For this review, take the finished solid that the model builds, in its own axes (mm). A direction names the side the tool comes from. Round coordinates to 2 decimals unless told otherwise and drop trailing zeros. Write each loop counter-clockwise with the first axis right and the second up, starting at its lowest first coordinate (ties: lowest second). Pieces come first, ordered by that corner, then holes. Notation, with made-up numbers: M 79,65.5 L 128,65.5 A33 ccw 128,97.5 Z; hole C 85.5,11 d2. An arc over 180 degrees is marked long. Answer in a Markdown table with one row per item.
```python
from build123d import *

# Parameters (mm, degrees)
SKETCH1_R           = 2.5
BOSS_EXTRUDE1_DEPTH = 2.5


with BuildPart() as part:
    # Sketch1 → Boss-Extrude1 (new body)
    with BuildSketch(Plane(origin=(0, 0, -1.25), x_dir=(-1, 0, 0), z_dir=(0, 0, -1))):
        with BuildLine():
            Line((-1.337750611, -12.7), (75.946, -12.7))
            Line((75.946, -12.7), (82.296, -6.35))
            Line((82.296, -6.35), (82.296, 6.35))
            Line((82.296, 6.35), (75.946, 12.7))
            Line((75.946, 12.7), (57.193204579, 12.7))
            ThreePointArc((57.193204579, 12.7), (55.429269089, 13.235083981), (54.259887063, 14.659980102))
            Line((54.259887063, 14.659980102), (48.733705431, 28.001362746))
            ThreePointArc((48.733705431, 28.001362746), (48.553029681, 29.835794416), (49.421958916, 31.461446674))
            Line((49.421958916, 31.461446674), (62.682187725, 44.721675483))
            Line((62.682187725, 44.721675483), (62.682187725, 53.701931604))
            Line((62.682187725, 53.701931604), (53.701931604, 62.682187725))
            Line((53.701931604, 62.682187725), (44.721675483, 62.682187725))
            Line((44.721675483, 62.682187725), (-9.92618865, 8.034323593))
            Line((-9.92618865, 8.034323593), (-1.337750611, -12.7))
        make_face()
        with Locations((12.7, 0)):
            Circle(SKETCH1_R, mode=Mode.SUBTRACT)
        with Locations((25.4, 0)):
            Circle(SKETCH1_R, mode=Mode.SUBTRACT)
        with Locations((38.1, 0)):
            Circle(SKETCH1_R, mode=Mode.SUBTRACT)
        with Locations((50.8, 0)):
            Circle(SKETCH1_R, mode=Mode.SUBTRACT)
        Circle(SKETCH1_R, mode=Mode.SUBTRACT)
        with Locations((76.2, 0)):
            Circle(SKETCH1_R, mode=Mode.SUBTRACT)
        with Locations((63.5, 0)):
            Circle(SKETCH1_R, mode=Mode.SUBTRACT)
        with Locations((53.881536726, 53.881536726)):
            Circle(SKETCH1_R, mode=Mode.SUBTRACT)
        with Locations((44.901280605, 44.901280605)):
            Circle(SKETCH1_R, mode=Mode.SUBTRACT)
        with Locations((35.921024484, 35.921024484)):
            Circle(SKETCH1_R, mode=Mode.SUBTRACT)
        with Locations((26.940768363, 26.940768363)):
            Circle(SKETCH1_R, mode=Mode.SUBTRACT)
        with Locations((17.960512242, 17.960512242)):
            Circle(SKETCH1_R, mode=Mode.SUBTRACT)
        with Locations((8.980256121, 8.980256121)):
            Circle(SKETCH1_R, mode=Mode.SUBTRACT)
    extrude(amount=-BOSS_EXTRUDE1_DEPTH)


solid = part.part
```
Q1. For probe 1 along Y at (x, z) = (-25.4, 0.7); probe 2 along Y at (x, z) = (-7.5, 0.1); probe 3 along Y at (x, z) = (-46, 0.05), list the stretches that pass through material, from the lowest coordinate up.
Found:
| item | result |
|---|---|
| probe 1 | -12.7 to -2.5, 2.5 to 24.97, 28.91 to 43.36 |
| probe 2 | -12.7 to 6.97, 10.99 to 25.46 |
| probe 3 | -12.7 to 42.66, 47.15 to 62.68 |
Q2. Take a section at A-A (y = 0). State how many separate pieces and enclosed holes the cut face has, then the cut area to 3 significant figures.
Found:
| item | result |
|---|---|
| separate pieces | 8 |
| enclosed holes | 0 |
| area | 135 mm² |
Q3. Mouldability with a two-part tool opening along Y and no side actions: class faces 3 (the face through (-55.96, 38, -0.02)), 4 (the face through (-36, 17, -1.25)), 5 (the face through (-17.78, 35.74, -0.02)) as +Y half, -Y half, draft (parallel to the pull), parting line (faces both ways), or undercut.
Found:
| item | result |
|---|---|
| face 3 | undercut |
| face 4 | draft |
| face 5 | +Y half |
Q4. Take a section at D-D (x = -12.7). State the section outline as (y, z) points.
Found:
| item | result |
|---|---|
| outline | M -12.7,-1.25 L -2.5,-1.25 L -2.5,1.25 L -12.7,1.25 Z; M 2.5,-1.25 L 30.66,-1.25 L 30.66,1.25 L 2.5,1.25 Z |
Q5. Take a section at B-B (x = 0). State the section outline as (y, z) points, then the cut area to 3 significant figures.
Found:
| item | result |
|---|---|
| outline | M -12.7,-1.25 L -2.5,-1.25 L -2.5,1.25 L -12.7,1.25 Z; M 2.5,-1.25 L 17.96,-1.25 L 17.96,1.25 L 2.5,1.25 Z |
| area | 64.2 mm² |
Q6. Machinability: for faces 1 (the face through (-36, 17, 1.25)), 2 (the face through (-51.535, 21.237, -0.018)), which of the approach directions +Z, -Z, +X, -X, +Y, -Y give a long, thin tool a straight path to every point of the face, cutting with its end or side? Answer none if there is none.
Found:
| item | result |
|---|---|
| face 1 | +Z, +X, -X, +Y, -Y |
| face 2 | +Z, -Z, -X |
Q7. Insertion check: P1, Ø6, axis at x = -63.5, y = 0, coming from the +Z side; P2, Ø0.8, axis at y = 48.5, z = 0, coming from the -X side. Each pin has a flat end and moves straight along its axis. Give the tip position at first contact, or say it passes through.
Found:
| item | result |
|---|---|
| P1 | z = 1.25 |
| P2 | x = -62.68 |
